Design review of the part built by this model. Coordinates are the model's own, in mm. A direction names the side the tool comes from. Coordinates: 2 decimals unless noted, no trailing zeros. Loops run counter-clockwise (first coordinate to the right, second up) from the corner with the lowest first, then second, coordinate; pieces in that order, holes last. Notation, with made-up numbers: (4.25, 43.5) - (26.25, 43.5) arc R19 ccw to (26.25, 58.5) - close; hole circle Ø7 at (-37.75, -12.75). An arc over 180 degrees is marked (long way). Answer in a Markdown table with one row per item. Add a question column.
(1) Clearance check with a flat-ended pin moving along its axis: pin 1 (1.9 mm diameter, centred on x = -1, y = -1, fed in from +Z). State where the tip first meets the part, or that it passes through.
(2) We need section B-B, the plane y = 0. Write out the cut boundary in (x, z).
(3) We need section C-C, the plane z = 4.5. Write out the cut boundary in (x, y), plus the area to 3 significant figures.
(4) To check wall thickness, follow L1, parallel to X at y = -1.8, z = 2.75; L2, parallel to Z at x = -1.9, y = -0.5; L3, parallel to Y at x = 0.65, z = 5.5. State the ranges of each line that lie inside material, in increasing order. Write a range as [from, to].
(5) We need section D-D, the plane y = -1.5. Write out the cut boundary in (x, z).
(6) For faces 1 (the face through (-2.75, 0, 3)), 2 (the face through (0.04, -1.25, 6.09)), 3 (the face through (-0.04, -1.25, -2.46)), list the 3-axis set-ups (+Z, -Z, +X, -X, +Y, -Y) from which the entire face can be reached by the end or side of a thin tool; tool diameter is ignored.
(7) We need section A-A, the plane x = 0. Write out the cut boundary in (y, z), plus the area to 3 significant figures.
Autodesk Inventor part; units mm, degrees
ref_plane "YZ Plane" through (0, 0, 0) normal (1, 0, 0) x (0, 1, 0)
ref_plane "XZ Plane" through (0, 0, 0) normal (0, 1, 0) x (-1, 0, 0)
ref_plane "XY Plane" through (0, 0, 0) normal (0, 0, 1) x (1, 0, 0)
sketch "Sketch1" plane through (0, 0, 0) normal (0, 0, 1) x (1, 0, 0)
  circle A0 centre (0, 0) radius 1.25
  circle A1 centre (0, 0) radius 2.75
  line L0 (-1.75, 2.75) -> (1.75, 2.75)
  line L1 (2.75, 1.75) -> (2.75, -1.75)
  line L2 (1.75, -2.75) -> (-1.75, -2.75)
  line L3 (-2.75, -1.75) -> (-2.75, 1.75)
  arc A2 (-1.75, 2.75) -> (-2.75, 1.75) centre (-1.75, 1.75) ccw
  arc A3 (2.75, 1.75) -> (1.75, 2.75) centre (1.75, 1.75) ccw
  arc A4 (1.75, -2.75) -> (2.75, -1.75) centre (1.75, -1.75) ccw
  arc A5 (-2.75, -1.75) -> (-1.75, -2.75) centre (-1.75, -1.75) ccw
  line L4 (-2.75, 1) -> (2.75, 1)
  point P0 (-2.75, 0)
  point P1 (0, -2.75)
  point P2 (0.75, 1)
  point P3 (-0.75, 1)
  dimension "d0" = 2.5
  dimension "d1" = 5.5
  dimension "d2" = 1
  dimension "d3" = 1
  dimension "d4" = 1
  dimension "d11" = 1
extrude "Extrusion1" add sketch "Sketch1" against normal blind 5 contours A0 L4 picked at (0.7457, -0.3378)
extrude "Extrusion2" add sketch "Sketch1" along normal blind 5.1 contours A0 L4 | A0 L4 A1 | L4 L1 A1 | A1 L3 L4 | L1 A4 L2 A1 | A1 L2 A5 L3 picked at (0.7457, -0.3378) picked at (2.227, -0.204)
extrude "Extrusion3" add sketch "Sketch1" along normal blind 7.1 contours A0 L4 picked at (0.7457, -0.3378)
properties part number "rpi_base_front_3DPrint"
Responses:
| question | item | result |
|---|---|---|
| 1 | pin 1 | stops at z = 7.1 |
| 2 | outline | (-2.75, 0) - (-1.25, 0) - (-1.25, -5) - (1.25, -5) - (1.25, 0) - (2.75, 0) - (2.75, 5.1) - (1.25, 5.1) - (1.25, 7.1) - (-1.25, 7.1) - (-1.25, 5.1) - (-2.75, 5.1) - close |
| 3 | outline | (-2.75, -1.75) arc R1 ccw to (-1.75, -2.75) - (1.75, -2.75) arc R1 ccw to (2.75, -1.75) - (2.75, 1) - (-2.75, 1) - close |
| 3 | area | 20.2 mm2 |
| 4 | L1 | x = [-2.75, 2.75] |
| 4 | L2 | z = [0, 5.1] |
| 4 | L3 | y = [-1.07, 1] |
| 5 | outline | (-2.75, 0) - (2.75, 0) - (2.75, 5.1) - (-2.75, 5.1) - close |
| 6 | face 1 | +Z, -Z, -X, +Y, -Y |
| 6 | face 2 | +Z |
| 6 | face 3 | -Z |
| 7 | outline | (-2.75, 0) - (-1.25, 0) - (-1.25, -5) - (1, -5) - (1, 7.1) - (-1.25, 7.1) - (-1.25, 5.1) - (-2.75, 5.1) - close |
| 7 | area | 34.9 mm2 |
